Here's how the part is built. I have some questions about the finished solid (model axes, mm). Round coordinates to 2 decimals unless told otherwise and drop trailing zeros. Loops run counter-clockwise (first coordinate to the right, second up) from the corner with the lowest first, then second, coordinate; pieces in that order, holes last. Notation, with made-up numbers: M 15,-26 L 22,-26 A26 cw 22,1 Z; hole C 38,13.25 d2. An arc over 180 degrees is marked long. Answer as a JSON object with one key per item and string values.
from build123d import *

# Parameters (mm, degrees)
CROQUIS1_R              = 2.5
CROQUIS1_R_2            = 2.55
CROQUIS1_R_3            = 3.15
SALIENTE_EXTRUIR1_DEPTH = 3


with BuildPart() as part:
    # Croquis1 → Saliente-Extruir1 (new body)
    with BuildSketch(Plane.XY):
        with BuildLine():
            Line((35, 77.5), (-35, 77.5))
            ThreePointArc((-35, 77.5), (-42.071067812, 74.571067812), (-45, 67.5))
            Line((-45, 67.5), (-45, -67.5))
            ThreePointArc((-45, -67.5), (-42.071067812, -74.571067812), (-35, -77.5))
            Line((-35, -77.5), (35, -77.5))
            ThreePointArc((35, -77.5), (42.071067812, -74.571067812), (45, -67.5))
            Line((45, -67.5), (45, 67.5))
            ThreePointArc((45, 67.5), (42.071067812, 74.571067812), (35, 77.5))
        make_face()
        with Locations((17.5, 62.325)):
            Circle(CROQUIS1_R, mode=Mode.SUBTRACT)
        with Locations(Location((17.5, -62.325, 0), (0, 0, 180))):
            Circle(CROQUIS1_R, mode=Mode.SUBTRACT)
        with Locations((-17.5, -62.325)):
            Circle(CROQUIS1_R, mode=Mode.SUBTRACT)
        with Locations(Location((-17.5, 62.325, 0), (0, 0, 180))):
            Circle(CROQUIS1_R, mode=Mode.SUBTRACT)
        with Locations((0, 10)):
            Circle(CROQUIS1_R_2, mode=Mode.SUBTRACT)
        with Locations(Location((0, -10, 0), (0, 0, 180))):
            Circle(CROQUIS1_R_2, mode=Mode.SUBTRACT)
        with Locations((-25, 34)):
            Circle(CROQUIS1_R_3, mode=Mode.SUBTRACT)
        with Locations(Location((25, 34, 0), (0, 0, 180))):
            Circle(CROQUIS1_R_3, mode=Mode.SUBTRACT)
    extrude(amount=SALIENTE_EXTRUIR1_DEPTH)


solid = part.part
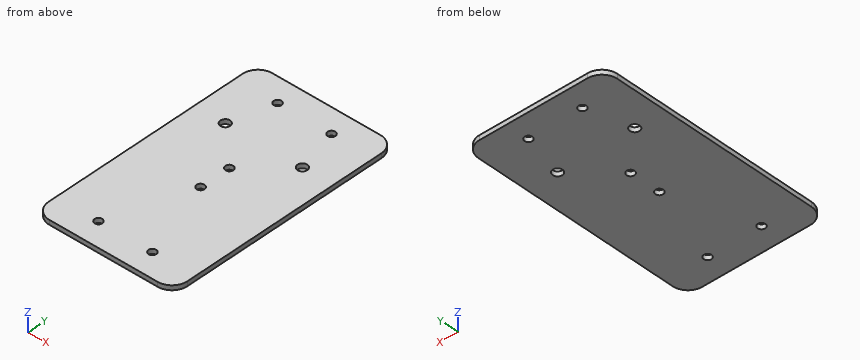
Item 1: For P1, Ø1.5, axis at x = -10.5, y = -25, coming from the -Z side, with a flat end and sliding along its axis, tell me the tip position at first contact or that it passes through.
Solution:
{"P1": "stops at z = 0"}
Item 2: I want a section at B-B on x = -25. List the corners of the cut face in (y, z) for me, plus the area to 3 significant figures.
Solution:
{"outline": "M -77.5,0 L 30.85,0 L 30.85,3 L -77.5,3 Z; M 37.15,0 L 77.5,0 L 77.5,3 L 37.15,3 Z", "area": "446 mm2"}
Item 3: I want a section at D-D on z = 1.35. Count the separate pieces of the cut face and the enclosed holes in it, plus the area to 3 significant figures.
Solution:
{"separate pieces": "1", "enclosed holes": "8", "area": "13,700 mm2"}
Item 4: If I drill on L1, parallel to Y at x = 17.5, z = 1.4 (3 decimals); L2, parallel to Y at x = 0, z = 0.6; L3, parallel to Y at x = 25, z = 2.05, over which ranges is the centre line in solid material (lowest first)? Write a range as from..to.
Solution:
{"L1": "y = -77.5..-64.825, -59.825..59.825, 64.825..77.5", "L2": "y = -77.5..-12.55, -7.45..7.45, 12.55..77.5", "L3": "y = -77.5..30.85, 37.15..77.5"}
Item 5: I want a section at A-A on y = -10. List the corners of the cut face in (x, z) for me.
Solution:
{"outline": "M -45,0 L -2.55,0 L -2.55,3 L -45,3 Z; M 2.55,0 L 45,0 L 45,3 L 2.55,3 Z"}
Item 6: I want a section at C-C on x = 17.5. List the corners of the cut face in (y, z) for me (3 decimals), plus the area to 3 significant figures.
Solution:
{"outline": "M -77.5,0 L -64.825,0 L -64.825,3 L -77.5,3 Z; M -59.825,0 L 59.825,0 L 59.825,3 L -59.825,3 Z; M 64.825,0 L 77.5,0 L 77.5,3 L 64.825,3 Z", "area": "435 mm2"}
